The model under review builds one solid part; all positions refer to its coordinate system, in mm. A direction names the side the tool comes from. Round coordinates to 2 decimals unless told otherwise and drop trailing zeros. Write each loop counter-clockwise with the first axis right and the second up, starting at its lowest first coordinate (ties: lowest second). Pieces come first, ordered by that corner, then holes.
Item 1: Add section B-B (z = 2.4). Give the boundary of the cut face in (x, y), plus the area to 3 significant figures.
Item 2: Add section A-A (x = -12.5). Give the boundary of the cut face in (y, z).
Item 3: Add section C-C (x = 0). Give the boundary of the cut face in (y, z).
Item 4: To check wall thickness, follow L1, parallel to Y at x = 0, z = 4.7; L2, parallel to Z at x = -0.5, y = 12; L3, parallel to X at y = -4, z = 4.25. State the ranges of each line that lie inside material, in increasing order.
Item 5: Machinability: for faces 4 (the face through (4.66, 4.9, 1.48)), 5 (the face through (-7, -5, 3)), which of the approach directions +Z, -Z, +X, -X, +Y, -Y give a long, thin tool a straight path to every point of the face, cutting with its end or side? Answer none if there is none.
Item 6: Clearance check with flat-ended pins moving along their axes: pin 1 Ø1.5 at (y, z) = (9, 1) entering from -X; pin 2 Ø3 at (y, z) = (-8, 4) entering from -X; pin 3 Ø2 at (x, z) = (-6, 4) entering from +Y. State where each tip first meets the part, or that it passes through.
Item 7: Add section D-D (y = -1.5). Give the boundary of the cut face in (x, z), plus the area to 3 significant figures.
Item 8: Draft analysis for pull direction Y (two halves, no side actions). For faces 1 (the face through (-6.199, -8.097, 4.479)), 2 (the face through (0, 0, 0)), 3 (the face through (-11, 0, 1)), state which applies: +Y half, -Y half, draft (parallel to the pull), parting line (faces both ways), or undercut.
```python
from build123d import *

# Parameters (mm, degrees)
F0_R     = 11
F0_R_2   = 1.25
F1_DEPTH = 3
F2_R     = 1.25
F2_R_2   = 2.5
F3_DEPTH = 3
F4_R     = 2.5
F5_DEPTH = 5


with BuildPart() as f1:
    # F0 (on Top) → F1 (new body)
    with BuildSketch(Plane.XY):
        Circle(F0_R)
        with Locations((-5.656854, -5.656854)):
            Circle(F0_R_2, mode=Mode.SUBTRACT)
        with Locations((5.656854, -5.656854)):
            Circle(F0_R_2, mode=Mode.SUBTRACT)
        with Locations((-5.656854, 5.656854)):
            Circle(F0_R_2, mode=Mode.SUBTRACT)
        with Locations((5.656854, 5.656854)):
            Circle(F0_R_2, mode=Mode.SUBTRACT)
    extrude(amount=F1_DEPTH)

    # F2 (on face) → F3 (join)
    with BuildSketch(Plane.XY.offset(3)):
        with BuildLine():
            ThreePointArc((-15.233871, 9.264706), (-13.2379, 0), (-15.233871, -9.264706))
            ThreePointArc((-15.233871, -9.264706), (-13.793453, -13.20684), (-9.821429, -11.85102))
            ThreePointArc((-9.821429, -11.85102), (-6.25, -9.65238), (-2.678571, -11.85102))
            ThreePointArc((-2.678571, -11.85102), (1.293453, -13.20684), (2.733871, -9.264706))
            ThreePointArc((2.733871, -9.264706), (0.7379, 0), (2.733871, 9.264706))
            ThreePointArc((2.733871, 9.264706), (1.293453, 13.20684), (-2.678571, 11.85102))
            ThreePointArc((-2.678571, 11.85102), (-6.25, 9.65238), (-9.821429, 11.85102))
            ThreePointArc((-9.821429, 11.85102), (-13.793453, 13.20684), (-15.233871, 9.264706))
        make_face()
        with Locations((-12.5, -10.5)):
            Circle(F2_R, mode=Mode.SUBTRACT)
        with Locations((0, -10.5)):
            Circle(F2_R, mode=Mode.SUBTRACT)
        with Locations((-5.656854, -5.656854)):
            Circle(F2_R_2, mode=Mode.SUBTRACT)
        with Locations((-12.5, 10.5)):
            Circle(F2_R, mode=Mode.SUBTRACT)
        with Locations((-5.656854, 5.656854)):
            Circle(F2_R_2, mode=Mode.SUBTRACT)
        with Locations((0, 10.5)):
            Circle(F2_R, mode=Mode.SUBTRACT)
    extrude(amount=F3_DEPTH)

    # F4 (on face) → F5 (cut)
    with BuildSketch(Plane(origin=(0, 0, 3), x_dir=(1, 0, 0), z_dir=(0, 0, -1))):
        with Locations((0, 10.5)):
            Circle(F4_R)
        with Locations((0, -10.5)):
            Circle(F4_R)
    extrude(amount=F5_DEPTH, mode=Mode.SUBTRACT)


solid = f1.part
```
Numbers:
1. outline: (-2.49, -10.71) arc R2.5 cw (long way) to (2.49, -10.71) arc R11 ccw to (2.49, 10.71) arc R2.5 cw (long way) to (-2.49, 10.71) arc R11 ccw to start; hole circle Ø2.5 at (-5.66, -5.66); hole circle Ø2.5 at (-5.66, 5.66); hole circle Ø2.5 at (5.66, -5.66); hole circle Ø2.5 at (5.66, 5.66)
1. area: 337 mm2
2. outline: (-13.5, 3) - (-11.75, 3) - (-11.75, 6) - (-13.5, 6) - close; (-9.25, 3) - (9.25, 3) - (9.25, 6) - (-9.25, 6) - close; (11.75, 3) - (13.5, 3) - (13.5, 6) - (11.75, 6) - close
3. outline: (-13.5, 3) - (-11.75, 3) - (-11.75, 6) - (-13.5, 6) - close; (-9.25, 3) - (-8, 3) - (-8, 0) - (8, 0) - (8, 3) - (9.25, 3) - (9.25, 6) - (-9.25, 6) - close; (11.75, 3) - (13.5, 3) - (13.5, 6) - (11.75, 6) - close
4. L1: y = -13.5 to -11.75, -9.25 to 9.25, 11.75 to 13.5
4. L2: z = 3 to 6
4. L3: x = -13.6 to -7.53, -3.78 to 1.1
5. face 4: +Z, -Z
5. face 5: +Z
6. pin 1: stops at x = -7.28
6. pin 2: stops at x = -15.33
6. pin 3: stops at y = 9.85
7. outline: (-13.29, 3) - (-10.9, 3) - (-10.9, 0) - (10.9, 0) - (10.9, 3) - (0.79, 3) - (0.79, 6) - (-13.29, 6) - close
7. area: 108 mm2
8. face 1: undercut
8. face 2: draft
8. face 3: parting line
